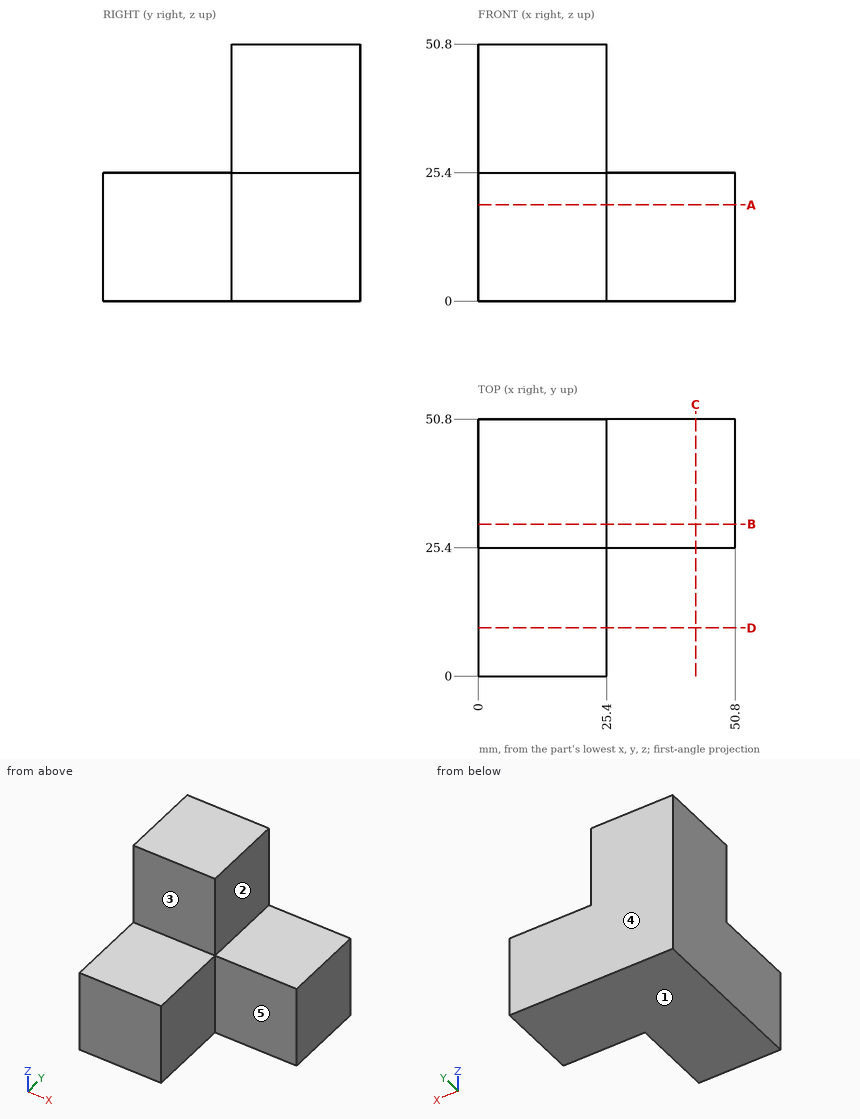
Geometry check sheet. Reference: drawing and pictorial views, mm from the part's lowest x, y, z. A direction names the side the tool comes from. Round coordinates to 2 decimals unless told otherwise and drop trailing zeros. Order: outer loops, then holes, each group sorted by start corner. A loop starts at its lowest first (then second) coordinate and runs counter-clockwise, first axis right, second up. Notation, with made-up numbers: M 23.5,-30 L 38.5,-30 A20 ccw 38.5,-24 Z; hole C -4.75,34 d2. An arc over 180 degrees is marked long. One line per item, written item: value. Start each with the question number.
1. Scan lines: line 1 along X through (y, z) = (10, 3.5); line 2 along Y through (x, z) = (46.5, 22). Record each from-to range of solid material in increasing order.
2. Section check B-B on y = 30. Enter the section's corners in (x, z), and give its area (3 significant figures).
3. Section check C-C on x = 43. Enter the section's corners in (y, z).
4. Section check D-D on y = 9.5. Enter the section's corners in (x, z), and give its area (3 significant figures).
5. Access from +Z, -Z, +X, -X, +Y, -Y to the whole of each face (thin tool, end or side, straight path). Record for the marked faces 1, 2, 3, 4 and 5.
6. Gauge pin test, flat ends, axial feed: P1, Ø12.5, axis at x = 10.5, y = 16, coming from the +Z side; P2, Ø7.5, axis at y = 16.5, z = 18, coming from the +X side; P3, Ø12.5, axis at x = 9.5, z = 40, coming from the -Y side. Record the tip position at first contact, or that the pin passes through.
7. Section check A-A on z = 19. Enter the section's corners in (x, y), and give its area (3 significant figures).
Results found:
1. line 1: 0 to 25.4
1. line 2: 25.4 to 50.8
2. outline: M 0,0 L 50.8,0 L 50.8,25.4 L 25.4,25.4 L 25.4,50.8 L 0,50.8 Z
2. area: 1,940 mm^2
3. outline: M 25.4,0 L 50.8,0 L 50.8,25.4 L 25.4,25.4 Z
4. outline: M 0,0 L 25.4,0 L 25.4,25.4 L 0,25.4 Z
4. area: 645 mm^2
5. face 1: -Z, +X, -X, +Y, -Y
5. face 2: +Z, +X, +Y, -Y
5. face 3: +Z, +X, -X, -Y
5. face 4: +Z, -Z, +X, -X, +Y
5. face 5: +Z, -Z, +X, -Y
6. P1: z = 25.4
6. P2: x = 25.4
6. P3: y = 25.4
7. outline: M 0,0 L 25.4,0 L 25.4,25.4 L 50.8,25.4 L 50.8,50.8 L 0,50.8 Z
7. area: 1,940 mm^2
